from build123d import *

# Parameters (mm, degrees)
SKETCH2_R               = 5
BOSS_EXTRUDE1_DEPTH     = 6
SKETCH3_R               = 2
CUT_EXTRUDE1_DEPTH      = 32.559467676
FILLET1_R               = 0.5
CUT_EXTRUDE2_DEPTH      = 31
CUT_EXTRUDE2_DEPTH_BACK = 31
SKETCH4_R               = 1


with BuildPart() as part:
    # Sketch1 → Revolve1 (revolve)
    with BuildSketch(Plane.XY):
        Polygon((-3.059401077, 20), (-0.75, 16), (0.75, 16), (3.059401077, 20), (4, 20), (4, 0), (-4, 0), (-4, 20), align=None)
    revolve(axis=Axis((4, 0, 0), (-1, 0, 0)))

    # Sketch2 → Boss-Extrude1 (add)
    with BuildSketch(Plane.ZY.offset(4)):
        with Locations(Location((0, 0, 0), (0, 0, 270))):
            Circle(SKETCH2_R)
    extrude(amount=BOSS_EXTRUDE1_DEPTH)

    # Sketch3 → Cut-Extrude1 (cut, through all)
    with BuildSketch(Plane.ZY.offset(10)):
        with Locations(Location((0, 0, 0), (0, 0, 270))):
            Circle(SKETCH3_R)
    extrude(amount=-CUT_EXTRUDE1_DEPTH, mode=Mode.SUBTRACT)

    # Fillet1
    fillet1_edges = [part.edges().sort_by_distance(p)[0] for p in [
        (-4, 5, 0),
        (-10, 5, 0),
    ]]
    fillet(fillet1_edges, radius=FILLET1_R)

    # Sketch4 → Cut-Extrude2 (cut, two sides: drawn at the far end of the back side and taken through both)
    with BuildSketch(Plane.XY.offset(-CUT_EXTRUDE2_DEPTH_BACK)):
        with Locations((-7, 0)):
            Circle(SKETCH4_R)
    extrude(amount=CUT_EXTRUDE2_DEPTH + CUT_EXTRUDE2_DEPTH_BACK, mode=Mode.SUBTRACT)


solid = part.part
Can you work these out from the model? Positions are in its coordinate system, mm. A direction names the side the tool comes from. Give positions to 0.01 mm unless a question says otherwise; leave off trailing zeros. Loops run counter-clockwise (first coordinate to the right, second up) from the corner with the lowest first, then second, coordinate; pieces in that order, holes last. Notation, with made-up numbers: (74, -25.5) - (131, -25.5) arc R12 cw to (131, -13.5) - close; hole circle Ø4 at (38, 57.25). An arc over 180 degrees is marked (long way). One line per item, written item: value.
(1) If we mould it in two halves opening along Y, with no side actions, what happens to faces 1 (the face through (-3.098, -1.847, -0.766)), 2 (the face through (-3.523, -4.336, 19.524)), 3 (the face through (-10, -1, -2))? For each: released by +Y, released by -Y, zero draft, split by the parting line, or undercut.
Verdict:
face 1: undercut
face 2: split by the parting line
face 3: zero draft
(2) If we section it at C-C, the plane x = -7: List the corners of the cut face in (y, z) for me, plus the area to 3 significant figures.
Verdict:
outline: (-1, -4.9) - (-1, -1.73) arc R2 cw to (-1, 1.73) - (-1, 4.9) arc R5 ccw to start; (1, -4.9) arc R5 ccw to (1, 4.9) - (1, 1.73) arc R2 cw to (1, -1.73) - close
area: 53.8 mm^2
(3) I need wall thicknesses on line 1 along Z through (x, y) = (0, 0); line 2 along X through (y, z) = (0, 4.2); line 3 along X through (y, z) = (-9, -3). Which ranges of each line are inside material? Lowest first, please.
Verdict:
line 1: -16 to -2, 2 to 16
line 2: -10 to -8, -6 to 4
line 3: -4 to 4
(4) If we section it at D-D, the plane x = -1.25: List the corners of the cut face in (y, z) for me, plus the area to 3 significant figures.
Verdict:
outline: circle Ø33.73 at (0, 0); hole circle Ø4 at (0, 0)
area: 881 mm^2
(5) If we section it at B-B, the plane y = 0: State how many separate pieces and enclosed holes the cut face has, plus the area to 3 significant figures.
Verdict:
separate pieces: 4
enclosed holes: 0
area: 282 mm^2
(6) On a 3-axis mill with a long thin cutter (end or side, diameter ignored), from which of +Z, -Z, +X, -X, +Y, -Y can I reach the whole of each face in a straight line? I mean faces 4 (the face through (-4, -4, 4)), 5 (the face through (0.01, -3.47, 15.62)), 6 (the face through (3.536, -4.336, 19.524)). Say none if no direction works.
Verdict:
face 4: -X
face 5: none
face 6: +X, -X
(7) I'm going to push flat-ended pins straight in: pin 1 (2.5 mm diameter, centred on x = -7, y = 0, fed in from +Z); pin 2 (8 mm diameter, centred on y = 11.5, z = 14.5, fed in from -X); pin 3 (5 mm diameter, centred on x = 0, z = -3, fed in from -Y). Where does each tip first touch, or does it pass through?
Verdict:
pin 1: z = 5
pin 2: x = -4
pin 3: y = -18.81
(8) If we section it at A-A, the plane z = 0: List the corners of the cut face in (x, y) for me.
Verdict:
outline: (-10, -4.5) arc R0.5 ccw to (-9.5, -5) - (-4.5, -5) arc R0.5 cw to (-4, -5.5) - (-4, -20) - (-3.06, -20) - (-0.75, -16) - (0.75, -16) - (3.06, -20) - (4, -20) - (4, -2) - (-10, -2) - close; (-10, 2) - (4, 2) - (4, 20) - (3.06, 20) - (0.75, 16) - (-0.75, 16) - (-3.06, 20) - (-4, 20) - (-4, 5.5) arc R0.5 cw to (-4.5, 5) - (-9.5, 5) arc R0.5 ccw to (-10, 4.5) - close
